```python
from build123d import *

# Parameters (mm, degrees)
F3_R     = 1.2
F3_R_2   = 35
F4_DEPTH = 3


with BuildPart() as f1:
    # F0 (on Right) → F1 (revolve)
    with BuildSketch(Plane.YZ):
        Polygon((2, 35), (-3, 35), (-3, 34), (1, 31), (2, 31), align=None)
    revolve(axis=Axis((0, 1.602868, 0), (0, -1, 0)))

    # F3 (on offset) → F4 (join)
    with BuildSketch(Plane.XZ.offset(1)):
        Polygon((-15, -36), (36, -36), (36, 36), (-36, 36), (-36, -15), align=None)
        with Locations((28, -28)):
            Circle(F3_R, mode=Mode.SUBTRACT)
        with Locations((-28, 28)):
            Circle(F3_R, mode=Mode.SUBTRACT)
        Circle(F3_R_2, mode=Mode.SUBTRACT)
        with Locations((28, 28)):
            Circle(F3_R, mode=Mode.SUBTRACT)
    extrude(amount=-F4_DEPTH)


solid = f1.part
```
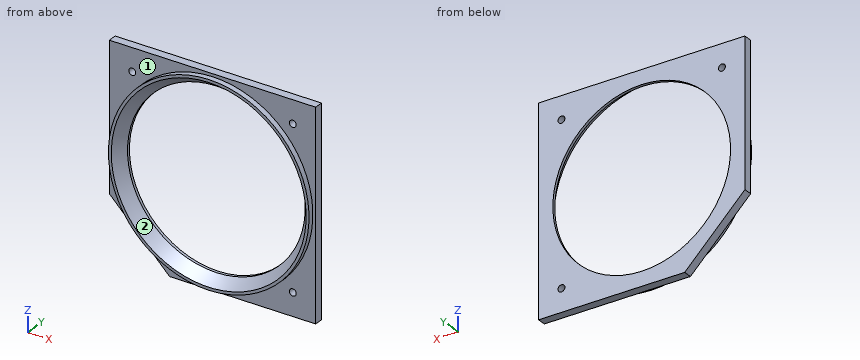
Input: part model. Units: mm. Frame: model coordinates. Face numbers are marked on the shaded views. Give positions to 0.01 mm unless a question says otherwise; leave off trailing zeros. Loops run counter-clockwise (first coordinate to the right, second up) from the corner with the lowest first, then second, coordinate; pieces in that order, holes last.
1) Section query C-C on z = 28. Count the separate pieces of the cut face and the enclosed holes in it, and give its area (3 significant figures).
A:
separate pieces: 4
enclosed holes: 0
area: 128 mm2
2) Section query A-A on z = 0. Return the cut outline in (x, y), and give its area (3 significant figures).
A:
outline: (-36, -1) - (-35, -1) - (-35, -3) - (-34, -3) - (-31, 1) - (-31, 2) - (-36, 2) - close; (31, 1) - (34, -3) - (35, -3) - (35, -1) - (36, -1) - (36, 2) - (31, 2) - close
area: 34.0 mm2
3) Contact query for flat-ended pins moving along their axis: pin 1 (3 mm diameter, centred on x = -28, z = 28, fed in from -Y); pin 2 (8 mm diameter, centred on x = -26.5, z = -2, fed in from -Y); pin 3 (1 mm diameter, centred on y = -2, z = 1, fed in from -X). Output: stop coordinate, or through.
A:
pin 1: stops at y = -1
pin 2: passes through
pin 3: stops at x = -35
4) Mould query, pull axis Z, two halves, no side actions, for the marked faces 1 and 2. Classes: released by +Z, released by -Z, zero draft, split by the parting line, or undercut.
A:
face 1: zero draft
face 2: undercut
5) Line query: L1, parallel to Z at x = -28, y = -0.4; L2, parallel to Z at x = 28, y = -0.05; L3, parallel to Z at x = 28, y = 0.4. Output: solid intervals per line, ascending.
A:
L1: z = -23 to -15.59, 15.59 to 26.8, 29.2 to 36
L2: z = -36 to -29.2, -26.8 to -15.05, 15.05 to 26.8, 29.2 to 36
L3: z = -36 to -29.2, -26.8 to -14.32, 14.32 to 26.8, 29.2 to 36
6) Section query B-B on x = 0. Return the cut outline in (y, z).
A:
outline: (-3, -35) - (-1, -35) - (-1, -36) - (2, -36) - (2, -31) - (1, -31) - (-3, -34) - close; (-3, 34) - (1, 31) - (2, 31) - (2, 36) - (-1, 36) - (-1, 35) - (-3, 35) - close
